from build123d import *

# Parameters (mm, degrees)
BOSS_EXTRUDE1_DEPTH = 2.54
SKETCH2_W           = 3.175
SKETCH2_H           = 7.366
BOSS_EXTRUDE2_DEPTH = 3.175
SKETCH3_W           = 3.175
SKETCH3_H           = 7.366
BOSS_EXTRUDE4_DEPTH = 10.668
SKETCH4_W           = 13.335
SKETCH4_H           = 7.366
BOSS_EXTRUDE5_DEPTH = 3.175


with BuildPart() as part:
    # Sketch1 → Boss-Extrude1 (new body)
    with BuildSketch(Plane(origin=(0, 0, 0), x_dir=(0, 0, -1), z_dir=(1, 0, 0))):
        Polygon((-47.389657734, -29.937142578), (-21.989657734, -29.937142578), (-21.989657734, -17.237142578), (16.110342266, 5.622857422), (21.714787013, 5.622857422), (21.714787013, 12.988857422), (2.987008932, 12.988857422), (-47.389657734, -17.237142578), align=None)
    extrude(amount=BOSS_EXTRUDE1_DEPTH)

    # Sketch2 → Boss-Extrude2 (add)
    with BuildSketch(Plane(origin=(2.54, 0, 0), x_dir=(0, 0, -1), z_dir=(1, 0, 0))):
        Polygon((16.110342266, 5.622857422), (21.714787013, 5.622857422), (21.714787013, 12.988857422), (11.554787013, 12.988857422), (11.554787013, 5.622857422), align=None)
        with Locations((9.967287013, 9.305857422)):
            Rectangle(SKETCH2_W, SKETCH2_H)
    extrude(amount=BOSS_EXTRUDE2_DEPTH)

    # Sketch3 → Boss-Extrude4 (add)
    with BuildSketch(Plane(origin=(5.715, 0, 0), x_dir=(0, 0, -1), z_dir=(1, 0, 0))):
        with Locations((20.127287013, 9.305857422)):
            Rectangle(SKETCH3_W, SKETCH3_H)
    extrude(amount=BOSS_EXTRUDE4_DEPTH)

    # Sketch4 → Boss-Extrude5 (add)
    with BuildSketch(Plane(origin=(16.383, 0, 0), x_dir=(0, 0, -1), z_dir=(1, 0, 0))):
        with Locations((15.047287013, 9.305857422)):
            Rectangle(SKETCH4_W, SKETCH4_H)
    extrude(amount=BOSS_EXTRUDE5_DEPTH)


solid = part.part
Work out the finished part from the listing and answer in its coordinate system (mm). A direction names the side the tool comes from. Round coordinates to 2 decimals unless told otherwise and drop trailing zeros. Loops run counter-clockwise (first coordinate to the right, second up) from the corner with the lowest first, then second, coordinate; pieces in that order, holes last. Notation, with made-up numbers: (49, -13) - (100, -13) arc R20 ccw to (100, 10) - close; hole circle Ø6 at (41, 87). An arc over 180 degrees is marked (long way). One line per item, written item: value.
Q1. Straight lines are drawn through the part: probe 1 along Z at (x, y) = (18.75, 10); probe 2 along X at (y, z) = (-15, 37); probe 3 along Z at (x, y) = (12.25, 11). For each, find the intervals that lie inside material, in ascending order.
Check values:
probe 1: -21.71 to -8.38
probe 2: 0 to 2.54
probe 3: -21.71 to -18.54
Q2. The mould has two halves that part along X. Classify faces 4 (the flat face through (5, 12.989, -14)), 5 (the flat face through (19.558, 9, -15)), 6 (the flat face through (16.383, 9, -13)): +X half, -X half, draft (parallel to the pull), parting line (faces both ways), or undercut.
Check values:
face 4: draft
face 5: +X half
face 6: undercut
Q3. Find section C-C on y = 8.5. Give the vertices of the cut face in (x, z) (3 decimals), and give its area (3 significant figures).
Check values:
outline: (0, -21.715) - (19.558, -21.715) - (19.558, -8.38) - (16.383, -8.38) - (16.383, -18.54) - (5.715, -18.54) - (5.715, -8.38) - (2.54, -8.38) - (2.54, 4.494) - (0, 4.494) - close
area: 185 mm2
Q4. Find section A-A on y = -19. Give the vertices of the cut face in (x, z), and give its area (3 significant figures).
Check values:
outline: (0, 21.99) - (2.54, 21.99) - (2.54, 47.39) - (0, 47.39) - close
area: 64.5 mm2
Q5. Find section B-B on x = 13.5. Give the vertices of the cut face in (y, z).
Check values:
outline: (5.62, -21.71) - (12.99, -21.71) - (12.99, -18.54) - (5.62, -18.54) - close
Q6. For faces 1 (the flat face through (11, 9, -18.54)), 2 (the flat face through (1, -24, 21.99)), 3 (the flat face through (18, 9, -8.38)), determine the directions among +Z, -Z, +X, -X, +Y, -Y from which every point of the face is accessible in a straight line to the end or side of a thin tool.
Check values:
face 1: +Z, +Y, -Y
face 2: -Z, +X, -X, -Y
face 3: +Z, +X, +Y, -Y
Q7. Each of these flat-tipped pins is pushed along its axis until it touches: pin 1 Ø1.5 at (x, z) = (2.5, -1) entering from -Y; pin 2 Ø2.5 at (x, y) = (17.5, 8.5) entering from +Z; pin 3 Ø1.3 at (x, y) = (1, -21.5) entering from -Z; pin 4 Ø6 at (y, z) = (1, 17) entering from -X. Where does it stop, or does it pass through?
Check values:
pin 1: y = -3.89
pin 2: z = -8.38
pin 3: z = 21.99
pin 4: x = 0
